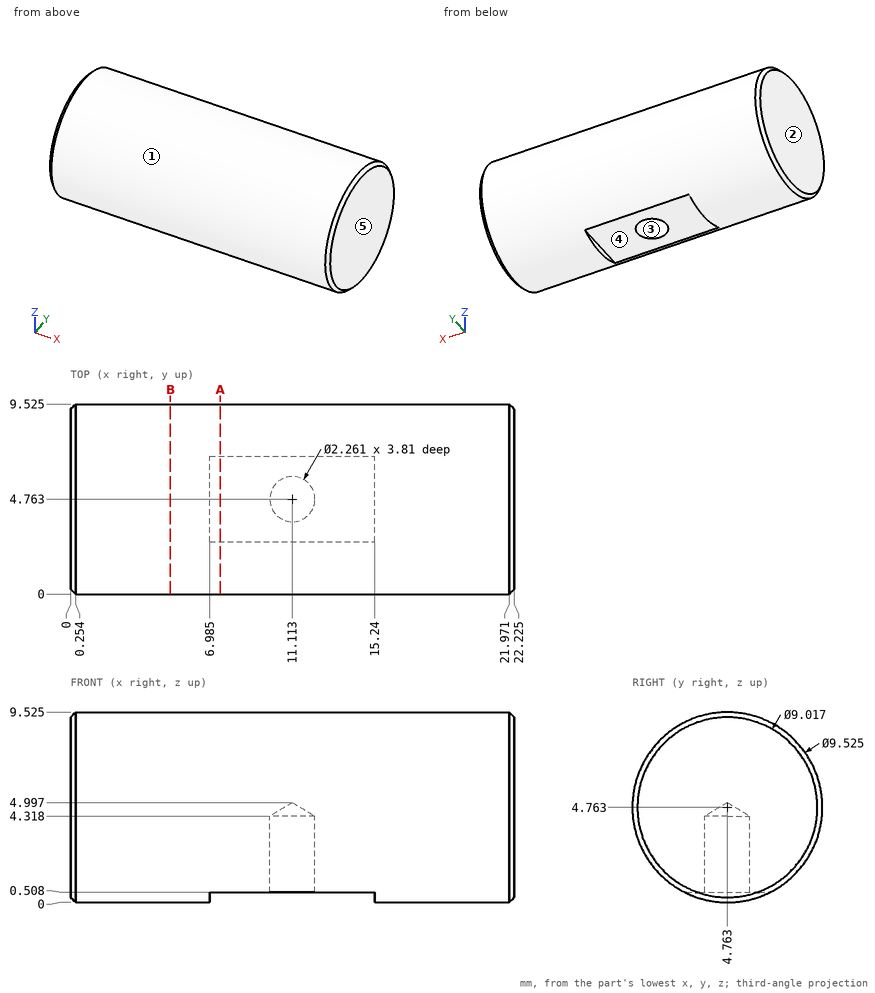
Geometry check sheet. Reference: drawing and pictorial views, mm from the part's lowest x, y, z. A direction names the side the tool comes from. Round coordinates to 2 decimals unless told otherwise and drop trailing zeros. Order: outer loops, then holes, each group sorted by start corner. A loop starts at its lowest first (then second) coordinate and runs counter-clockwise, first axis right, second up. Notation, with made-up numbers: (83, -9) -> (88, -9) arc R30 cw to (88, 18) -> close; hole circle Ø6 at (-13.5, -29). An arc over 180 degrees is marked (long way). One line per item, written item: value. Start each with the question number.
Q1. Mould release check, pull along Y, two halves, no side actions. Record for the marked faces 1, 2 and 3: pulls with the +Y half, pulls with the -Y half, needs draft (parallel to the pull), parting line crosses it, or undercut.
Q2. Gauge pin test, flat ends, axial feed: pin 1 Ø2 at (y, z) = (8, 7.5) entering from -X; pin 2 Ø4 at (x, y) = (18.5, 8.5) entering from +Z; pin 3 Ø1.3 at (x, y) = (13, 3.5) entering from -Z; pin 4 Ø2 at (x, z) = (12, 3.5) entering from -Y. Record the tip position at first contact, or that the pin passes through.
Q3. Thickness scan on line 1 (Y direction, x = 9.25, z = 8) (1 decimal); line 2 (Z direction, x = 8.25, y = 4.25); line 3 (Z direction, x = 15.75, y = 7.5) (1 decimal). Record the ranges inside material, lowest first.
Q4. Cross-section at B-B (x = 5). Record the boundary of the cut face in (y, z) (1 decimal).
Q5. Cross-section at A-A (x = 7.5). Record the boundary of the cut face in (y, z) (1 decimal), and give its area (3 significant figures).
Q6. Set-up check for the marked faces 4 and 5: record each of +Z, -Z, +X, -X, +Y, -Y from which the full face is reachable in a straight line by a thin tool's end or side.
Completed:
1. face 1: parting line crosses it
1. face 2: needs draft
1. face 3: undercut
2. pin 1: stops at x = 0
2. pin 2: stops at z = 9.2
2. pin 3: stops at z = 0.51
2. pin 4: stops at y = 0.01
3. line 1: y = 1.3 to 8.3
3. line 2: z = 0.51 to 9.5
3. line 3: z = 0.9 to 8.7
4. outline: circle Ø9.5 at (4.8, 4.8)
5. outline: (2.6, 0.5) -> (6.9, 0.5) arc R4.8 ccw (long way) to start
5. area: 69.8 mm²
6. face 4: -Z, +Y, -Y
6. face 5: +Z, -Z, +X, +Y, -Y
